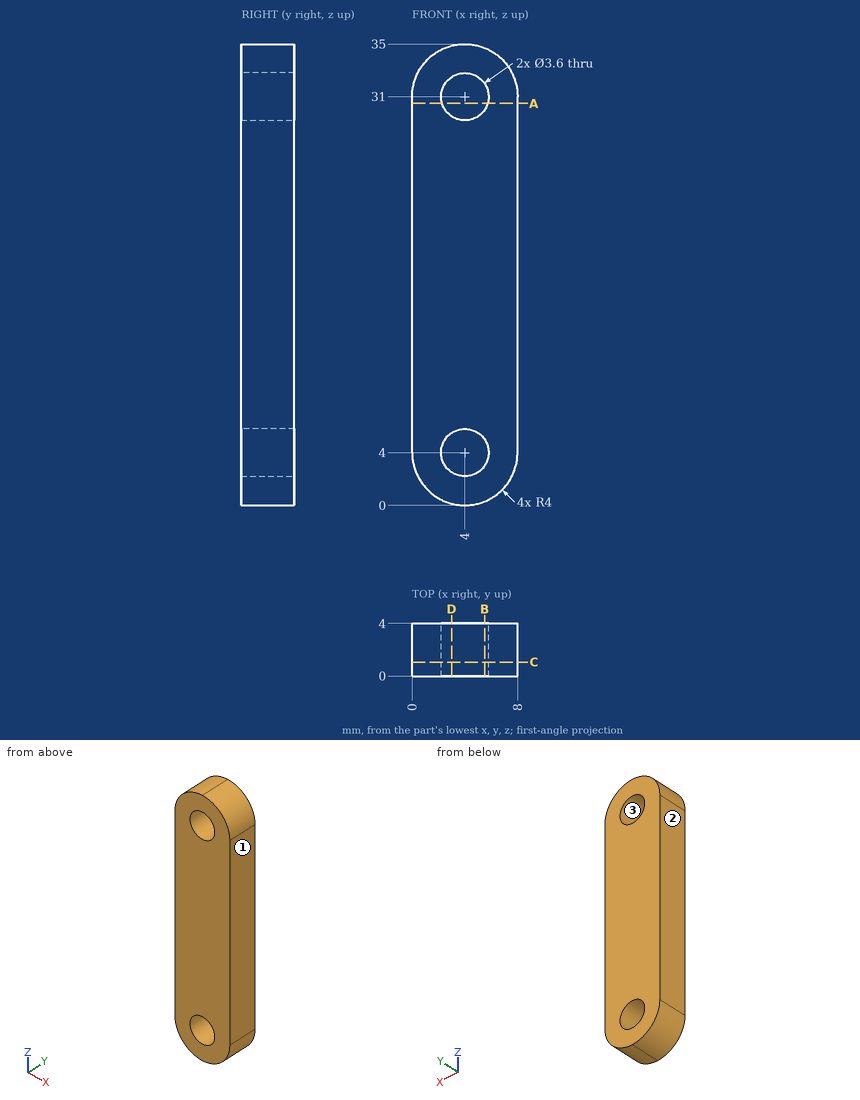
The figure shows three views and two pictorial views of one solid part (mm, origin at its lowest corner). Answer the questions. Round coordinates to 2 decimals unless told otherwise and drop trailing zeros. Write each loop counter-clockwise with the first axis right and the second up, starting at its lowest first coordinate (ties: lowest second). Pieces come first, ordered by that corner, then holes. Notation, with made-up numbers: (24, -24) -> (55, -24) arc R28 cw to (55, 4) -> close; hole circle Ø11 at (-39, 41.5). An arc over 180 degrees is marked (long way). Write each question's results on one line, items separated by ' | '.
Q1. Determine the mould class of the marked faces 1, 2 and 3 for opening direction X: released by +X, released by -X, zero draft, split by the parting line, or undercut.
Data:
face 1: released by +X | face 2: released by -X | face 3: undercut
Q2. Flat-ended cylindrical pins translate along their axes: P1, Ø3, axis at x = 4, z = 31, coming from the +Y side; P2, Ø3, axis at x = 4, z = 24.5, coming from the -Y side; P3, Ø1.5, axis at x = 1.5, y = 0.5, coming from the -Z side. Find the tip coordinate at first contact, or state that the pin passes through.
Data:
P1: through | P2: y = 0 | P3: z = 0.4
Q3. Section A-A, the plane z = 30.5 is taken. Write down the section's boundary in (x, y).
Data:
outline: (0, 0) -> (2.27, 0) -> (2.27, 4) -> (0, 4) -> close; (5.73, 0) -> (8, 0) -> (8, 4) -> (5.73, 4) -> close
Q4. Straight lines are drawn through the part: line 1 along X through (y, z) = (1.55, 4); line 2 along Z through (x, y) = (3.75, 3.3); line 3 along Z through (x, y) = (2.5, 2.7) (1 decimal). For each, find the intervals that lie inside material, in ascending order. Write a range as [from, to].
Data:
line 1: [0, 2.2], [5.8, 8] | line 2: [0.01, 2.22], [5.78, 29.22], [32.78, 34.99] | line 3: [0.3, 3], [5, 30], [32, 34.7]
Q5. Section B-B, the plane x = 5.5 is taken. Write down the section's boundary in (y, z) (3 decimals), then the cut area to 3 significant figures.
Data:
outline: (0, 0.292) -> (4, 0.292) -> (4, 3.005) -> (0, 3.005) -> close; (0, 4.995) -> (4, 4.995) -> (4, 30.005) -> (0, 30.005) -> close; (0, 31.995) -> (4, 31.995) -> (4, 34.708) -> (0, 34.708) -> close | area: 122 mm^2
Q6. Section C-C, the plane y = 1.05 is taken. Give the number of separate pieces and of enclosed holes in the cut face, then the cut area to 3 significant figures.
Data:
separate pieces: 1 | enclosed holes: 2 | area: 246 mm^2
Q7. Section D-D, the plane x = 3 is taken. Write down the section's boundary in (y, z).
Data:
outline: (0, 0.13) -> (4, 0.13) -> (4, 2.5) -> (0, 2.5) -> close; (0, 5.5) -> (4, 5.5) -> (4, 29.5) -> (0, 29.5) -> close; (0, 32.5) -> (4, 32.5) -> (4, 34.87) -> (0, 34.87) -> close
